Read the model definition and answer for the solid it produces. Units are mm, in the model's axes. Face numbers are marked on the shaded views. A direction names the side the tool comes from. Coordinates: 2 decimals unless noted, no trailing zeros. Loops run counter-clockwise (first coordinate to the right, second up) from the corner with the lowest first, then second, coordinate; pieces in that order, holes last. Notation, with made-up numbers: (7.5, 20) -> (64.5, 20) arc R6 ccw to (64.5, 28) -> close; hole circle Ø6 at (79.25, 61.5). An arc over 180 degrees is marked (long way). Answer as a JSON object with one key per item and string values. Group by question number.
1) Section D-D, the plane x = 25.4 is taken. Give the vertices of the cut face in (y, z), plus the area to 3 significant figures.
2) Section A-A, the plane x = -42.38 is taken. Give the vertices of the cut face in (y, z).
3) Flat-ended cylindrical pins translate along their axes: P1, Ø2.5, axis at x = -42.38, z = -42.38, coming from the -Y side; P2, Ø8, axis at x = 10.5, z = -8.5, coming from the +Y side. Find the tip coordinate at first contact, or state that the pin passes through.
4) Section B-B, the plane z = 42.38 is taken. Give the vertices of the cut face in (x, y), plus the area to 3 significant figures.
5) Consider probe 1 along Z at (x, y) = (-42.38, 0.75); probe 2 along X at (y, z) = (36, -44.5); probe 3 along Z at (x, y) = (36, 33.5). Determine where each line is inside the solid, lowest interval first. Write a range as [from, to].
6) Section C-C, the plane y = 31 is taken. Give the vertices of the cut face in (x, z), plus the area to 3 significant figures.
7) Determine the mould class of the marked faces 3, 4, 5 and 6 for opening direction Z: released by +Z, released by -Z, zero draft, split by the parting line, or undercut.
8) Which of the six approach directions +Z, -Z, +X, -X, +Y, -Y give full straight-line access (tool end or side, diameter ignored) to the marked faces 1 and 2?
Autodesk Inventor part; units mm, degrees
ref_plane "YZ Plane" through (0, 0, 0) normal (1, 0, 0) x (0, 1, 0)
ref_plane "XZ Plane" through (0, 0, 0) normal (0, 1, 0) x (-1, 0, 0)
ref_plane "XY Plane" through (0, 0, 0) normal (0, 0, 1) x (1, 0, 0)
sketch "Sketch1" plane through (0, 0, 0) normal (0, 1, 0) x (-1, 0, 0)
  line L0 (-63.5, 50.8) -> (63.5, 50.8)
  line L1 (63.5, 50.8) -> (63.5, -50.8)
  line L2 (63.5, -50.8) -> (-63.5, -50.8)
  line L3 (-63.5, -50.8) -> (-63.5, 50.8)
  line L4 (-63.5, 50.8) -> (63.5, -50.8) construction
  line L5 (63.5, 50.8) -> (-63.5, -50.8) construction
  point P0 (0, 0)
  dimension "d0" = 127
  dimension "d1" = 101.6
extrude "Extrusion1" add sketch "Sketch1" along normal blind 1.016
sketch "Sketch2" plane through (0, 1.016, 0) normal (0, 1, 0) x (1, 0, 0)
  line L0 (63.5, 50.8) -> (-63.5, 50.8)
  line L1 (63.5, -50.8) -> (-63.5, -50.8)
  line L2 (-63.5, -50.8) -> (-63.5, 50.8)
  line L3 (-63.5, 50.8) -> (63.5, 50.8)
  line L4 (63.5, 50.8) -> (63.5, -50.8)
  line L5 (63.5, -50.8) -> (-63.5, 50.8) construction
  line L6 (-63.5, -50.8) -> (63.5, 50.8) construction
  line L7 (62.992, -50.292) -> (-62.992, -50.292)
  line L8 (-62.992, -50.292) -> (-62.992, 50.292)
  line L9 (-62.992, 50.292) -> (62.992, 50.292)
  line L10 (62.992, 50.292) -> (62.992, -50.292)
  line L11 (62.992, -50.292) -> (-62.992, 50.292) construction
  line L12 (-62.992, -50.292) -> (62.992, 50.292) construction
  point P0 (0, 0)
  dimension "d4" = 125.984
  dimension "d5" = 100.584
extrude "Extrusion2" add sketch "Sketch2" along normal blind 50.8
sketch "Sketch3" plane through (-62.992, 1.016, -50.292) normal (0, 0, 1) x (1, 0, 0)
  line L0 (0, 0) -> (0, 50.8)
  circle A0 centre (37.592, 25.4) radius 2.0828
  circle A1 centre (88.392, 25.4) radius 2.0828
  point P0 (62.992, -1.016)
  dimension "d10" = 4.1656
  dimension "d12" = 4.1656
extrude "Extrusion3" cut sketch "Sketch3" against normal through all
sketch "Sketch4" plane through (-62.992, 1.016, 50.292) normal (1, 0, 0) x (0, 0, -1)
  line L0 (0, 0) -> (0, 50.8)
  line L1 (0, 17.581) -> (50.292, 17.581)
  circle A0 centre (50.292, 17.581) radius 3.175
  point P0 (50.292, -1.016)
  dimension "d15" = 6.35
extrude "Extrusion4" cut sketch "Sketch4" against normal through all
sketch "Sketch5" plane through (62.992, 1.016, -50.292) normal (-1, 0, 0) x (0, 0, 1)
  line L0 (0, 0) -> (0, 50.8)
  line L1 (0, 19.05) -> (0.2921, 19.05)
  line L2 (0, 19.05) -> (0.2921, 19.05) construction
  line L3 (0.2921, 19.05) -> (16.1671, 19.05)
  line L4 (16.1671, 19.05) -> (49.5173, 19.05)
  line L5 (49.5173, 19.05) -> (20.9423, 19.05)
  line L6 (20.9423, 19.05) -> (49.5173, 19.05)
  line L7 (49.5173, 19.05) -> (78.0923, 19.05)
  circle A0 centre (78.0923, 19.05) radius 3.175
  circle A1 centre (49.5173, 19.05) radius 3.175
  circle A2 centre (16.1671, 19.05) radius 3.175
  point P0 (50.292, -1.016)
  dimension "d18" = 0.2921
  dimension "d19" = 0
  dimension "d20" = 15.875
  dimension "d21" = 33.3502
  dimension "d22" = 180
  dimension "d23" = 28.575
  dimension "d24" = 0
  dimension "d25" = 28.575
  dimension "d26" = 6.35
  dimension "d27" = 6.35
  dimension "d28" = 6.35
extrude "Extrusion5" cut sketch "Sketch5" against normal through all
sketch "Sketch6" plane through (0, 1.016, 0) normal (0, 1, 0) x (1, 0, 0)
  line L0 (-50, 50) -> (50, -50) construction
  line L1 (50, 50) -> (-50, -50) construction
  circle A0 centre (43.65, 42.38) radius 1.4224
  circle A1 centre (43.65, -42.38) radius 1.4224
  circle A2 centre (-42.38, -42.38) radius 1.4224
  circle A3 centre (-42.38, 42.38) radius 1.4224
  point P0 (0, 0)
  dimension "d31" = 100
  dimension "d32" = 100
  dimension "d38" = 2.8448
  dimension "d39" = 2.8448
  dimension "d40" = 2.8448
  dimension "d41" = 2.8448
extrude "Extrusion6" cut sketch "Sketch6" against normal through all
properties part number "563-AC-1404-5x4-Enclosure"
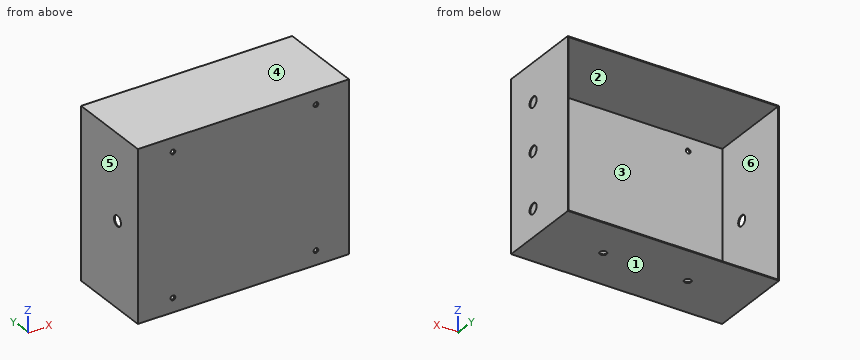
Determined:
{
 "1": {"outline": "(0, -50.8) -> (24.33, -50.8) -> (24.33, -50.29) -> (1.02, -50.29) -> (1.02, 50.29) -> (51.82, 50.29) -> (51.82, 50.8) -> (0, 50.8) -> close; (28.5, -50.8) -> (51.82, -50.8) -> (51.82, -50.29) -> (28.5, -50.29) -> close", "area": "153 mm²"},
 "2": {"outline": "(0, -50.8) -> (51.82, -50.8) -> (51.82, -50.29) -> (1.02, -50.29) -> (1.02, -43.8) -> (0, -43.8) -> close; (0, -40.96) -> (1.02, -40.96) -> (1.02, 40.96) -> (0, 40.96) -> close; (0, 43.8) -> (1.02, 43.8) -> (1.02, 50.29) -> (51.82, 50.29) -> (51.82, 50.8) -> (0, 50.8) -> close"},
 "3": {"P1": "through", "P2": "y = 1.02"},
 "4": {"outline": "(-63.5, 0) -> (-43.8, 0) -> (-43.8, 1.02) -> (-62.99, 1.02) -> (-62.99, 51.82) -> (-63.5, 51.82) -> close; (-40.96, 0) -> (42.23, 0) -> (42.23, 1.02) -> (-40.96, 1.02) -> close; (45.07, 0) -> (63.5, 0) -> (63.5, 51.82) -> (62.99, 51.82) -> (62.99, 1.02) -> (45.07, 1.02) -> close", "area": "175 mm²"},
 "5": {"probe 1": "[-50.8, -43.8], [-40.96, 40.96], [43.8, 50.8]", "probe 2": "[-63.5, -62.99], [62.99, 63.5]", "probe 3": "[-50.8, -50.29], [50.29, 50.8]"},
 "6": {"outline": "(-63.5, -50.8) -> (63.5, -50.8) -> (63.5, 50.8) -> (-63.5, 50.8) -> close; hole (-62.99, -50.29) -> (62.99, -50.29) -> (62.99, 50.29) -> (-62.99, 50.29) -> close", "area": "231 mm²"},
 "7": {"face 3": "undercut", "face 4": "released by +Z", "face 5": "zero draft", "face 6": "undercut"},
 "8": {"face 1": "-Z, +X, -X, +Y, -Y", "face 2": "+Y"}
}
